```python
from build123d import *

# Parameters (mm, degrees)
ESQUISSE1_W        = 5.72
ESQUISSE1_H        = 4.45
BOSS_EXTRU_1_DEPTH = 1.57
BOSS_EXTRU_2_START = -0.68
BOSS_EXTRU_2_DEPTH = 0.51
ESQUISSE4_W        = 12.7
ESQUISSE4_H        = 0.5
BOSS_EXTRU_3_DEPTH = 0.51


with BuildPart() as part:
    # Esquisse1 → Boss.-Extru.1 (new body)
    with BuildSketch(Plane.XY):
        with Locations((-1.64, 0)):
            Rectangle(ESQUISSE1_W, ESQUISSE1_H)
    extrude(amount=BOSS_EXTRU_1_DEPTH)

    # Esquisse2 → Révolution5 (revolve)
    with BuildSketch(Plane(origin=(0, 0, 0), x_dir=(1, 0, 0), z_dir=(0, 1, 0))):
        with BuildLine():
            Line((0, -0.81), (0, -2.33))
            ThreePointArc((0, -2.33), (0.76, -1.57), (0, -0.81))
        make_face()
    revolve(axis=Axis((0, 0, 0), (0, 0, 1)))

    # Esquisse3 → Boss.-Extru.2 (add)
    with BuildSketch(Plane.XY.offset(1.57).offset(BOSS_EXTRU_2_START)):
        Polygon((-4.5, 1.46), (-5.39, 1.46), (-5.39, 2.16), (-17.2, 2.16), (-17.2, 1.66), (-5.89, 1.66), (-5.89, 0.96), (-4.5, 0.96), align=None)
    boss_extru_2 = extrude(amount=-BOSS_EXTRU_2_DEPTH)

    # Symétrie1: Boss.-Extru.2 across plane
    add(boss_extru_2.mirror(Plane.ZX))

    # Esquisse4 → Boss.-Extru.3 (add)
    with BuildSketch(Plane.XY.offset(0.89)):
        with Locations((-10.85, 0)):
            Rectangle(ESQUISSE4_W, ESQUISSE4_H)
    extrude(amount=-BOSS_EXTRU_3_DEPTH)


solid = part.part
```
Verification items for the finished model (mm, model axes). A direction names the side the tool comes from. Give positions to 0.01 mm unless a question says otherwise; leave off trailing zeros. Order: outer loops, then holes, each group sorted by start corner. A loop starts at its lowest first (then second) coordinate and runs counter-clockwise, first axis right, second up. Notation, with made-up numbers: M 69,11 L 96,11 A23 ccw 96,35 Z; hole C -9.5,9 d1. An arc over 180 degrees is marked long. Answer in a Markdown table with one row per item. Add a question column.
Item 1: Section check A-A, the plane x = -15. Enter the section's corners in (y, z), and give its area (3 significant figures).
Item 2: Section check C-C, the plane z = 0.6. Enter the section's corners in (x, y) (3 decimals).
Item 3: Section check D-D, the plane x = -0.5. Enter the section's corners in (y, z) (3 decimals), and give its area (3 significant figures).
Item 4: Section check B-B, the plane y = -1.85. Enter the section's corners in (x, z), and give its area (3 significant figures).
Item 5: Tool access check on faces 1 (the flat face through (-11, 2, 0.89)), 2 (the flat face through (-11, 2, 0.38)), 3 (the flat face through (-2, -2.225, 1)). Record the directions out of +Z, -Z, +X, -X, +Y, -Y that give a thin tool (end or side, any length) a straight path to the whole face; none if there is none.
Item 6: Mould release check, pull along X, two halves, no side actions. Record for faces 4 (the flat face through (1.22, 0, 1)), 5 (the flat face through (-11, -2, 0.89)), 6 (the flat face through (-4.5, 0, 1.1)): released by +X, released by -X, zero draft, split by the parting line, or undercut.
Item 7: Gauge pin test, flat ends, axial feed: pin 1 (0.6 mm diameter, centred on x = -10.5, y = -1.5, fed in from +Z); pin 2 (1.3 mm diameter, centred on x = -10, y = -1.5, fed in from -Z). Record the tip position at first contact, or that the pin passes through.
Item 8: Scan lines: probe 1 along Y at (x, z) = (-9.25, 0.75); probe 2 along X at (y, z) = (-1.8, 0.45); probe 3 along X at (y, z) = (1.4, 0.5). Record each from-to range of solid material in increasing order. Write a range as from..to.
Filled sheet:
| question | item | result |
|---|---|---|
| 1 | outline | M -2.16,0.38 L -1.66,0.38 L -1.66,0.89 L -2.16,0.89 Z; M -0.25,0.38 L 0.25,0.38 L 0.25,0.89 L -0.25,0.89 Z; M 1.66,0.38 L 2.16,0.38 L 2.16,0.89 L 1.66,0.89 Z |
| 1 | area | 0.765 mm^2 |
| 2 | outline | M -17.2,-2.16 L -5.39,-2.16 L -5.39,-1.46 L -4.5,-1.46 L -4.5,-2.225 L 1.22,-2.225 L 1.22,2.225 L -4.5,2.225 L -4.5,1.46 L -5.39,1.46 L -5.39,2.16 L -17.2,2.16 L -17.2,1.66 L -5.89,1.66 L -5.89,0.96 L -4.5,0.96 L -4.5,0.25 L -17.2,0.25 L -17.2,-0.25 L -4.5,-0.25 L -4.5,-0.96 L -5.89,-0.96 L -5.89,-1.66 L -17.2,-1.66 Z |
| 3 | outline | M -2.225,0 L 2.225,0 L 2.225,1.57 L 0.572,1.57 A0.572 ccw -0.572,1.57 L -2.225,1.57 Z |
| 3 | area | 7.50 mm^2 |
| 4 | outline | M -17.2,0.38 L -5.39,0.38 L -5.39,0.89 L -17.2,0.89 Z; M -4.5,0 L 1.22,0 L 1.22,1.57 L -4.5,1.57 Z |
| 4 | area | 15.0 mm^2 |
| 5 | face 1 | +Z, -X, +Y, -Y |
| 5 | face 2 | -Z, -X, +Y, -Y |
| 5 | face 3 | +Z, -Z, +X, -X, -Y |
| 6 | face 4 | released by +X |
| 6 | face 5 | zero draft |
| 6 | face 6 | undercut |
| 7 | pin 1 | stops at z = 0.89 |
| 7 | pin 2 | stops at z = 0.38 |
| 8 | probe 1 | y = -2.16..-1.66, -0.25..0.25, 1.66..2.16 |
| 8 | probe 2 | x = -17.2..-5.39, -4.5..1.22 |
| 8 | probe 3 | x = -5.89..1.22 |
